Build history of the part. All positions in model axes, mm. Round coordinates to 2 decimals unless told otherwise and drop trailing zeros. Write each loop counter-clockwise with the first axis right and the second up, starting at its lowest first coordinate (ties: lowest second). Pieces come first, ordered by that corner, then holes.
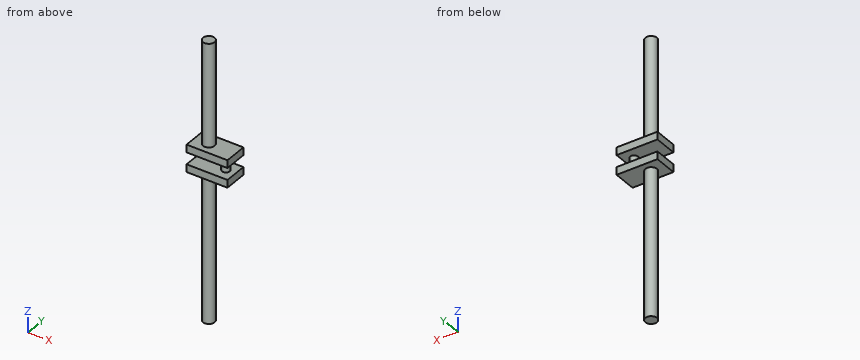
from build123d import *

# Parameters (mm, degrees)
SKETCH1_R           = 7.5
BOSS_EXTRUDE1_DEPTH = 180
SKETCH2_W           = 60
SKETCH2_H           = 25
CUT_EXTRUDE2_DEPTH  = 20
SKETCH3_W           = 52.918405924
SKETCH3_H           = 10
EXTRUDE_THIN1_DEPTH = 15
SKETCH4_R           = 5
BOSS_EXTRUDE2_DEPTH = 25


with BuildPart() as part:
    # Sketch1 → Boss-Extrude1 (new body, symmetric)
    with BuildSketch(Plane.XY):
        Circle(SKETCH1_R)
    extrude(amount=BOSS_EXTRUDE1_DEPTH, both=True)

    # Sketch2 → Cut-Extrude2 (cut, symmetric)
    with BuildSketch(Plane(origin=(0, 0, 0), x_dir=(1, 0, 0), z_dir=(0, 1, 0))):
        with Locations((14.409183819, -24.262804911)):
            Rectangle(SKETCH2_W, SKETCH2_H)
    extrude(amount=CUT_EXTRUDE2_DEPTH, both=True, mode=Mode.SUBTRACT)

    # Sketch3 → Extrude-Thin1 (add, symmetric)
    with BuildSketch(Plane(origin=(0, 0, 0), x_dir=(1, 0, 0), z_dir=(0, 1, 0))):
        with Locations((7.967689598, -16.457817956)):
            Rectangle(SKETCH3_W, SKETCH3_H)
        with Locations((7.967689598, -41.762804911)):
            Rectangle(SKETCH3_W, SKETCH3_H)
    extrude(amount=EXTRUDE_THIN1_DEPTH, both=True)

    # Sketch4 → Boss-Extrude2 (add)
    with BuildSketch(Plane.XY.offset(21.457817956)):
        with Locations((22.078448721, 0)):
            Circle(SKETCH4_R)
    extrude(amount=BOSS_EXTRUDE2_DEPTH)


solid = part.part
1) Slice it at B-B (y = -11). Write the cut outline in (x, z).
Results:
outline: (-18.49, 11.46) - (34.43, 11.46) - (34.43, 21.46) - (-18.49, 21.46) - close; (-18.49, 36.76) - (34.43, 36.76) - (34.43, 46.76) - (-18.49, 46.76) - close
2) Pin check, flat tips, straight feed: pin 1 Ø1.5 at (x, y) = (20, 3) entering from +Z; pin 2 Ø8 at (x, z) = (9.5, -43) entering from +Y; pin 3 Ø8 at (y, z) = (-6, 108) entering from -X. Stop position of each tip, or through.
Results:
pin 1: stops at z = 46.76
pin 2: stops at y = 5.1
pin 3: stops at x = -7.23
3) Wall check: L1, parallel to Z at x = -2, y = -13; L2, parallel to Z at x = 2.5, y = 1; L3, parallel to Z at x = 21, y = -3.5. Give the ranges that are in metal, low to high.
Results:
L1: z = 11.46 to 21.46, 36.76 to 46.76
L2: z = -180 to 21.46, 36.76 to 180
L3: z = 11.46 to 46.76
4) Slice it at A-A (x = 0). Write the cut outline in (y, z), plus the area to 3 significant figures.
Results:
outline: (-15, 11.46) - (-7.5, 11.46) - (-7.5, -180) - (7.5, -180) - (7.5, 11.46) - (15, 11.46) - (15, 21.46) - (-15, 21.46) - close; (-15, 36.76) - (15, 36.76) - (15, 46.76) - (7.5, 46.76) - (7.5, 180) - (-7.5, 180) - (-7.5, 46.76) - (-15, 46.76) - close
area: 5,470 mm2
5) Slice it at C-C (z = 128). Write the cut outline in (x, y).
Results:
outline: circle Ø15 at (0, 0)
